The listing builds one solid part. Answer for the finished solid, in the listing's coordinates (mm). Face numbers are marked on the shaded views. A direction names the side the tool comes from. Give positions to 0.01 mm unless a question says otherwise; leave off trailing zeros. Write each loop counter-clockwise with the first axis right and the second up, starting at its lowest first coordinate (ties: lowest second). Pieces come first, ordered by that corner, then holes. Notation, with made-up numbers: M 32.5,71 L 47.5,71 A25 ccw 47.5,97 Z; hole C -6,-22.75 d10. An arc over 180 degrees is marked long. Return JSON: item names as keys, results as strings.
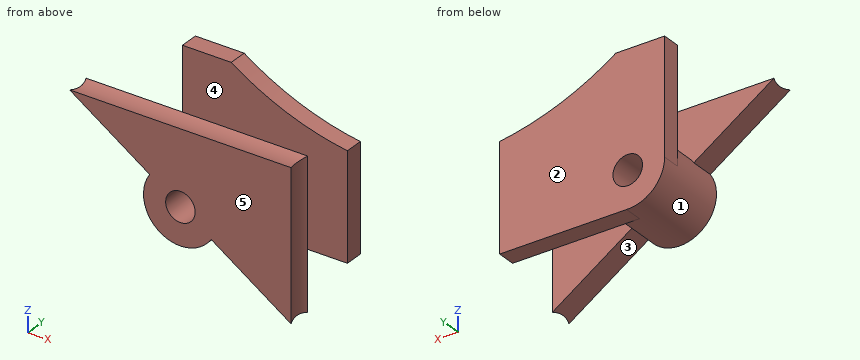
from build123d import *

# Parameters (mm, degrees)
BOSS_EXTRUDE1_DEPTH     = 6.35
SKETCH1_3_R             = 10
SKETCH1_3_R_2           = 4
BOSS_EXTRUDE2_DEPTH     = 20
CUT_EXTRUDE1_DEPTH      = 42.231056256
CUT_EXTRUDE1_DEPTH_BACK = 42.231056256
SKETCH3_R               = 7.768492306
CUT_EXTRUDE3_DEPTH      = 42.231056256
CUT_EXTRUDE3_DEPTH_BACK = 42.231056256
SKETCH4_R               = 12.223418735
BOSS_EXTRUDE3_START     = -5
BOSS_EXTRUDE3_DEPTH     = 5


with BuildPart() as part:
    # Sketch1 → Boss-Extrude1 (new body)
    with BuildSketch(Plane(origin=(0, 0, 0), x_dir=(1, 0, 0), z_dir=(0, 1, 0))):
        with BuildLine():
            Line((30, -20), (30, 20))
            Line((30, 20), (8.320502943, 5.547001962))
            ThreePointArc((8.320502943, 5.547001962), (9.570920265, 2.897841487), (10, 0))
            ThreePointArc((10, 0), (2.897841487, -9.570920265), (-8.320502943, -5.547001962))
            Line((-8.320502943, -5.547001962), (-30, -20))
            Line((-30, -20), (30, -20))
        make_face()
    extrude(amount=BOSS_EXTRUDE1_DEPTH)

    # Sketch1<3> → Boss-Extrude2 (add)
    # profile 1 of 3: a face of its own
    with BuildSketch(Plane(origin=(0, 0, 0), x_dir=(1, 0, 0), z_dir=(0, 1, 0))):
        with Locations(Location((0, 0, 0), (0, 0, 33.690067526))):
            Circle(SKETCH1_3_R)
        with Locations(Location((0, 0, 0), (0, 0, 270))):
            Circle(SKETCH1_3_R_2, mode=Mode.SUBTRACT)
    # profile 2 of 3: a face of its own
    with BuildSketch(Plane(origin=(0, 0, 0), x_dir=(1, 0, 0), z_dir=(0, 1, 0))):
        with BuildLine():
            ThreePointArc((10, 0), (9.570920265, 2.897841487), (8.320502943, 5.547001962))
            Line((8.320502943, 5.547001962), (3.328201177, 2.218800785))
            ThreePointArc((3.328201177, 2.218800785), (3.828368106, 1.159136595), (4, 0))
            ThreePointArc((4, 0), (1.159136595, -3.828368106), (-3.328201177, -2.218800785))
            Line((-3.328201177, -2.218800785), (-8.320502943, -5.547001962))
            ThreePointArc((-8.320502943, -5.547001962), (2.897841487, -9.570920265), (10, 0))
        make_face()
    # profile 3 of 3: a face of its own
    with BuildSketch(Plane(origin=(0, 0, 0), x_dir=(1, 0, 0), z_dir=(0, 1, 0))):
        with BuildLine():
            Line((3.328201177, 2.218800785), (8.320502943, 5.547001962))
            ThreePointArc((8.320502943, 5.547001962), (-5.547001962, 8.320502943), (-8.320502943, -5.547001962))
            Line((-8.320502943, -5.547001962), (-3.328201177, -2.218800785))
            ThreePointArc((-3.328201177, -2.218800785), (-2.218800785, 3.328201177), (3.328201177, 2.218800785))
        make_face()
    extrude(amount=BOSS_EXTRUDE2_DEPTH)

    # Sketch3 → Cut-Extrude1 (cut, two sides: drawn at the far end of the back side and taken through both)
    with BuildSketch(Plane.XY.offset(-CUT_EXTRUDE1_DEPTH_BACK)):
        with Locations((37.090052729, 3.175)):
            Circle(SKETCH3_R)
    extrude(amount=CUT_EXTRUDE1_DEPTH + CUT_EXTRUDE1_DEPTH_BACK, mode=Mode.SUBTRACT)

    # Sketch4 → Cut-Extrude3 (cut, two sides: drawn at the far end of the back side and taken through both)
    with BuildSketch(Plane(origin=(0, 0, 0), x_dir=(0, 0, -1), z_dir=(1, 0, 0)).offset(-CUT_EXTRUDE3_DEPTH_BACK)):
        with Locations((-31.803869729, 3.175)):
            Circle(SKETCH4_R)
    extrude(amount=CUT_EXTRUDE3_DEPTH + CUT_EXTRUDE3_DEPTH_BACK, mode=Mode.SUBTRACT)

    # Sketch5 → Boss-Extrude3 (add)
    with BuildSketch(Plane(origin=(0, 20, 0), x_dir=(1, 0, 0), z_dir=(0, 1, 0)).offset(BOSS_EXTRUDE3_START)):
        with BuildLine():
            Line((34.688363183, 9.995142945), (0.311636817, 9.995142945))
            ThreePointArc((0.311636817, 9.995142945), (7.18040278, 6.960015511), (10, 0))
            ThreePointArc((10, 0), (0, -10), (-10, 0))
            Line((-10, 0), (-10, -30.985714007))
            Line((-10, -30.985714007), (3.222370876, -30.985714007))
            ThreePointArc((3.222370876, -30.985714007), (18.272166371, -23.133524369), (34.688363183, -18.813604371))
            Line((34.688363183, -18.813604371), (34.688363183, 9.995142945))
        make_face()
    extrude(amount=BOSS_EXTRUDE3_DEPTH)


solid = part.part
Item 1: Find the intervals of material crossed by line 1 (Z direction, x = 0, y = 13.5); line 2 (Y direction, x = 25, z = 7); line 3 (X direction, y = 17, z = 16.5), in increasing order.
Geometry results:
{"line 1": "z = -10 to -4, 4 to 10", "line 2": "y = 0 to 6.35, 15 to 20", "line 3": "x = -10 to 34.69"}
Item 2: Given pin 1 Ø5.5 at (y, z) = (18, 16.5) entering from -X; pin 2 Ø4 at (x, y) = (21, 18) entering from -Z; pin 3 Ø4 at (y, z) = (2.5, 16) entering from +X, each flat-ended and moving along its own axis, determine where each tip first touches the part or whether it passes through.
Geometry results:
{"pin 1": "stops at x = -10", "pin 2": "stops at z = -10", "pin 3": "stops at x = 29.8"}
Item 3: A cutting plane is placed at A-A, the plane y = 18.75. Write down the section's boundary in (x, z), plus the area to 3 significant figures.
Geometry results:
{"outline": "M -10,0 A10 ccw 0.31,-10 L 34.69,-10 L 34.69,18.81 A76.08 cw 3.22,30.99 L -10,30.99 Z; hole C 0,0 d8", "area": "1,530 mm2"}
Item 4: A cutting plane is placed at C-C, the plane x = 20. Write down the section's boundary in (y, z) (3 decimals), plus the area to 3 significant figures.
Geometry results:
{"outline": "M 0,-13.333 L 6.35,-13.333 L 6.35,20 A12.223 cw 0,20 Z; M 15,-9.995 L 20,-9.995 L 20,22.489 L 15,22.489 Z", "area": "372 mm2"}
Item 5: Which of the six approach directions +Z, -Z, +X, -X, +Y, -Y give full straight-line access (tool end or side, diameter ignored) to the marked faces 1 and 2?
Geometry results:
{"face 1": "none", "face 2": "+Z, -Z, +X, -X, +Y"}
Item 6: Determine the mould class of the marked faces 3, 4 and 5 for opening direction Y: +Y half, -Y half, draft (parallel to the pull), parting line (faces both ways), or undercut.
Geometry results:
{"face 3": "draft", "face 4": "undercut", "face 5": "-Y half"}
